For this review, take the finished solid that the model builds, in its own axes (mm). Face numbers are marked on the shaded views. A direction names the side the tool comes from. Round coordinates to 2 decimals unless told otherwise and drop trailing zeros. Order: outer loops, then holes, each group sorted by start corner. A loop starts at its lowest first (then second) coordinate and runs counter-clockwise, first axis right, second up. Notation, with made-up numbers: (83.25, 59) - (115.25, 59) arc R21 cw to (115.25, 98) - close; hole circle Ø11 at (28.5, 29). An arc over 180 degrees is marked (long way). One line per question, with ' | ' between items.
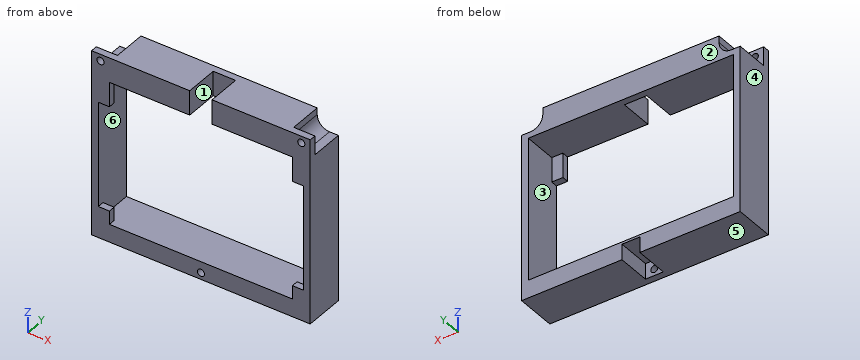
Autodesk Inventor part; units mm, degrees
ref_plane "YZ Plane" through (0, 0, 0) normal (1, 0, 0) x (0, 1, 0)
ref_plane "XZ Plane" through (0, 0, 0) normal (0, 1, 0) x (-1, 0, 0)
ref_plane "XY Plane" through (0, 0, 0) normal (0, 0, 1) x (1, 0, 0)
sketch "Szkic1" plane through (0, 0, 0) normal (0, 1, 0) x (-1, 0, 0)
  line L0 (0, 0) -> (-98, 0)
  line L1 (-98, 0) -> (-98, -83)
  line L2 (-98, -83) -> (0, -83)
  line L3 (0, -83) -> (0, 0)
  line L4 (-3, -11) -> (-95, -11)
  line L5 (-95, -11) -> (-95, -75)
  line L6 (-95, -75) -> (-3, -75)
  line L7 (-3, -75) -> (-3, -11)
  dimension "d0" = 83
  dimension "d1" = 98
  dimension "d2" = 92
  dimension "d3" = 3
  dimension "d4" = 8
  dimension "d5" = 64
extrude "Wyciągnięcie proste1" add sketch "Szkic1" along normal blind 18
sketch "Szkic2" plane through (0, 0, 0) normal (0, 0, 1) x (1, 0, 0)
  line L0 (0, 0) -> (49, 0) construction
  line L1 (49, 0) -> (49, 15) construction
  line L2 (44, 15) -> (54, 15)
  line L3 (44, 15) -> (44, 0)
  line L4 (44, 0) -> (54, 0)
  line L5 (54, 0) -> (54, 15)
  dimension "d8" = 15
  dimension "d9" = 49
  dimension "d64" = 10
sketch "Szkic3" plane through (0, 18, 0) normal (0, 1, 0) x (1, 0, 0)
  line L0 (0, 0) -> (0, 83) construction
  line L1 (0, 83) -> (49, 83) construction
  line L2 (49, 83) -> (49, 80) construction
  line L3 (49, 80) -> (49, 76) construction
  circle A0 centre (49, 80) radius 1.6
  line L4 (45, 76) -> (53, 76)
  line L5 (45, 76) -> (45, 83)
  line L6 (53, 76) -> (53, 83)
  line L7 (53, 83) -> (45, 83)
  dimension "d20" = 3
  dimension "d21" = 4
  dimension "d22" = 49
  dimension "d23" = 83
  dimension "d24" = 3.2
  dimension "d25" = 8
extrude "Wyciągnięcie proste3" cut sketch "Szkic3" against normal blind 15 contours A0 | L5 L7 L6 L4
extrude "Wyciągnięcie proste4" cut sketch "Szkic3" against normal through all contours A0
sketch "Szkic4" plane through (0, 18, 0) normal (0, 1, 0) x (1, 0, 0)
  line L0 (0, 0) -> (0, 3)
  line L1 (0, 3) -> (4, 3)
  circle A0 centre (4, 3) radius 1.6
  circle A1 centre (4, 3) radius 5.5
  line L2 (9.5, 3) -> (9.5, -5)
  line L3 (4, 8.5) -> (-4, 8.5)
  line L4 (-4, 8.5) -> (-4, -5)
  line L5 (-4, -5) -> (9.5, -5)
  line L6 (0, 0) -> (98, 0) construction
  line L7 (98, 0) -> (98, 3) construction
  line L8 (98, 3) -> (94, 3) construction
  circle A2 centre (94, 3) radius 1.6
  circle A3 centre (94, 3) radius 5.5
  line L9 (94, 8.5) -> (102, 8.5)
  line L10 (102, 8.5) -> (102, -5)
  line L11 (102, -5) -> (88.5, -5)
  line L12 (88.5, -5) -> (88.5, 3)
  dimension "d30" = 4
  dimension "d31" = 3
  dimension "d32" = 3.2
  dimension "d33" = 11
  dimension "d34" = 8
  dimension "d35" = 8
  dimension "d36" = 98
  dimension "d37" = 3
  dimension "d38" = 4
  dimension "d39" = 11
  dimension "d40" = 3.2
  dimension "d41" = 8
  dimension "d42" = 8
extrude "Wyciągnięcie proste5" cut sketch "Szkic4" against normal blind 15 contours A0 | A1 | L2 L5 L4 L3 A1 | A2 | A3 | A3 L9 L10 L11 L12
extrude "Wyciągnięcie proste6" cut sketch "Szkic4" against normal through all contours A0 | A2
sketch "Szkic5" plane through (0, 0, 0) normal (0, -1, 0) x (1, 0, 0)
  line L0 (0, 0) -> (0, -11) construction
  line L1 (0, -11) -> (0, -75) construction
  line L2 (0, -75) -> (3, -75) construction
  line L3 (0, -11) -> (3, -11) construction
  line L4 (0, 0) -> (98, 0) construction
  line L5 (98, 0) -> (98, -11) construction
  line L6 (98, -11) -> (95, -11) construction
  line L7 (98, -11) -> (98, -75) construction
  line L8 (98, -75) -> (95, -75) construction
  line L9 (3, -11) -> (8, -11)
  line L10 (8, -11) -> (8, -22)
  line L11 (8, -22) -> (3, -22)
  line L12 (3, -22) -> (3, -11)
  line L13 (3, -75) -> (8, -75)
  line L14 (8, -75) -> (8, -69)
  line L15 (8, -69) -> (3, -69)
  line L16 (3, -69) -> (3, -75)
  line L17 (95, -11) -> (90, -11)
  line L18 (90, -11) -> (90, -22)
  line L19 (90, -22) -> (95, -22)
  line L20 (95, -22) -> (95, -11)
  line L21 (95, -75) -> (90, -75)
  line L22 (90, -75) -> (90, -69)
  line L23 (90, -69) -> (95, -69)
  line L24 (95, -69) -> (95, -75)
  dimension "d47" = 3
  dimension "d48" = 3
  dimension "d49" = 11
  dimension "d50" = 64
  dimension "d51" = 98
  dimension "d52" = 11
  dimension "d53" = 3
  dimension "d54" = 3
  dimension "d55" = 64
  dimension "d56" = 11
  dimension "d57" = 5
  dimension "d58" = 6
  dimension "d59" = 5
  dimension "d60" = 6
  dimension "d61" = 11
extrude "Wyciągnięcie proste7" add sketch "Szkic5" against normal blind 3
extrude "Wyciągnięcie proste8" cut sketch "Szkic2" against normal blind 15
(1) We need section D-D on y = 4.75. State the section outline as (x, z) points, plus the area to 3 significant figures.
Output values:
outline: (0, -83) - (45, -83) - (45, -76) - (53, -76) - (53, -83) - (98, -83) - (98, -8.5) - (94, -8.5) arc R5.5 cw to (88.5, -3) - (88.5, 0) - (54, 0) - (54, -11) - (95, -11) - (95, -75) - (3, -75) - (3, -11) - (44, -11) - (44, 0) - (9.5, 0) - (9.5, -3) arc R5.5 cw to (4, -8.5) - (0, -8.5) - close | area: 1,930 mm^2
(2) We need section C-C on x = 49. State the section outline as (y, z) points.
Output values:
outline: (0, -83) - (3, -83) - (3, -81.6) - (0, -81.6) - close; (0, -78.4) - (3, -78.4) - (3, -76) - (18, -76) - (18, -75) - (0, -75) - close; (15, -11) - (18, -11) - (18, 0) - (15, 0) - close
(3) Mouldability with a two-part tool opening along X and no side actions: class the marked faces 4, 5 and 6 as released by +X, released by -X, zero draft, split by the parting line, or undercut.
Output values:
face 4: released by -X | face 5: zero draft | face 6: undercut
(4) For the marked faces 1, 2 and 3, list the 3-axis set-ups (+Z, -Z, +X, -X, +Y, -Y) from which the entire face can be reached by the end or side of a thin tool; tool diameter is ignored.
Output values:
face 1: +Z, -Y | face 2: +Z, -Z, +X, -X, +Y | face 3: +Y
(5) We need section B-B on z = -32.5. State the section outline as (x, y) points, plus the area to 3 significant figures.
Output values:
outline: (0, 0) - (3, 0) - (3, 18) - (0, 18) - close; (95, 0) - (98, 0) - (98, 18) - (95, 18) - close | area: 108 mm^2
(6) Insertion check: pin 1 (2.5 mm diameter, centred on x = 93.5, y = 1, fed in from +Z); pin 2 (1.2 mm diameter, centred on x = 1, y = 9, fed in from +Z); pin 3 (2.5 mm diameter, centred on x = 92, z = -70.5, fed in from +Y). Each pin has a flat end and moves straight along its axis. Give the tip position at first contact, or say it passes through.
Output values:
pin 1: z = 0 | pin 2: z = -8.5 | pin 3: y = 3
(7) We need section A-A on x = 29.5. State the section outline as (y, z) points.
Output values:
outline: (0, -83) - (18, -83) - (18, -75) - (0, -75) - close; (0, -11) - (18, -11) - (18, 0) - (0, 0) - close
(8) For probe 1 along Z at (x, y) = (94, 1.5); probe 2 along X at (y, z) = (1.6, -3); probe 3 along Z at (x, y) = (62, 6.5), list the stretches that pass through material, from the lowest coordinate up. Write a range as [from, to].
Output values:
probe 1: [-83, -69], [-22, -4.6], [-1.4, 0] | probe 2: [0, 2.4], [5.6, 44], [54, 92.4], [95.6, 98] | probe 3: [-83, -75], [-11, 0]
